Can you work these out from the model? Positions are in its coordinate system, mm. A direction names the side the tool comes from. Give positions to 0.01 mm unless a question says otherwise; leave off trailing zeros. Order: outer loops, then holes, each group sorted by start corner. A loop starts at its lowest first (then second) coordinate and runs counter-clockwise, first axis right, second up. Notation, with made-up numbers: (36.25, -33) - (53.25, -33) arc R8 ccw to (53.25, -20) - close; hole circle Ø6 at (-39.75, 82). An arc over 180 degrees is marked (long way). Answer as a JSON object with one key per item and string values.
```python
from build123d import *

# Parameters (mm, degrees)
BOSS_EXTRUDE1_DEPTH = 12.7
SKETCH2_R           = 1.1303
CUT_EXTRUDE1_DEPTH  = 10
SKETCH3_R           = 3.2639
CUT_EXTRUDE2_DEPTH  = 10


with BuildPart() as part:
    # Sketch1 → Boss-Extrude1 (new body)
    # profile 1 of 4: a face of its own
    with BuildSketch(Plane.XY):
        Polygon((-152.4, 0), (0, 0), (-114.3, -65.991135768), align=None)
        Polygon((-119.404432116, -6.35), (-31.030871047, -6.35), (-29.197783942, -9.525), (-95.477954744, -47.791874454), align=None, mode=Mode.SUBTRACT)
    # profile 2 of 4: a face of its own
    with BuildSketch(Plane.XY):
        Polygon((-165.1, 21.997045256), (-170.599261314, 18.822045256), (-157.899261314, -3.175), (-152.4, 0), align=None)
    # profile 3 of 4: a face of its own
    with BuildSketch(Plane.XY):
        Polygon((-157.899261314, -3.175), (-119.799261314, -69.166135768), (-114.3, -65.991135768), (-152.4, 0), align=None)
    # profile 4 of 4: a face of its own
    with BuildSketch(Plane.XY):
        Polygon((-107.099261314, -91.163181024), (-119.799261314, -69.166135768), (-114.3, -65.991135768), (-101.6, -87.988181024), align=None)
    extrude(amount=BOSS_EXTRUDE1_DEPTH)

    # Sketch2 → Cut-Extrude1 (cut)
    with BuildSketch(Plane(origin=(0, 0, 0), x_dir=(1, 0, 0), z_dir=(0, 1, 0))):
        with Locations(Location((-127, -6.35, 0), (0, 0, 180))):
            Circle(SKETCH2_R)
        with Locations(Location((-25.4, -6.35, 0), (0, 0, 180))):
            Circle(SKETCH2_R)
    extrude(amount=-CUT_EXTRUDE1_DEPTH, mode=Mode.SUBTRACT)

    # Sketch3 → Cut-Extrude2 (cut)
    with BuildSketch(Plane(origin=(-114.3, -65.991135768, 0), x_dir=(0, 0, -1), z_dir=(0.8660254037844342, 0.5000000000000079, 0))):
        with Locations(Location((-6.35, 88.9, 0), (0, 0, 90))):
            Circle(SKETCH3_R)
        with Locations(Location((-6.35, -12.7, 0), (0, 0, 90))):
            Circle(SKETCH3_R)
    extrude(amount=-CUT_EXTRUDE2_DEPTH, mode=Mode.SUBTRACT)


solid = part.part
```
Q1. I'm going to push flat-ended pins straight in: pin 1 Ø1.5 at (y, z) = (-15, 6.5) entering from -X; pin 2 Ø1.5 at (x, z) = (-57.5, 1.5) entering from -Y; pin 3 Ø1.5 at (y, z) = (-29.5, 7.5) entering from -X; pin 4 Ø3 at (x, y) = (-126.5, -64.5) entering from +Z. Where does each tip first touch, or does it pass through?
Recorded:
{"pin 1": "stops at x = -151.51", "pin 2": "stops at y = -33.63", "pin 3": "stops at x = -143.13", "pin 4": "passes through"}
Q2. Which directions (+Z, -Z, +X, -X, +Y, -Y) give clear straight access to the entire face, cutting with the end or side of a thin tool? Please do faces 5 (the face through (-77, 0, 6)), 6 (the face through (-109.45, -74.39, 9.08)), 7 (the face through (-167.811, 20.432, 6.261)), 8 (the face through (-30.127, -7.915, 6.261)).
Recorded:
{"face 5": "+Z, -Z, +X, +Y", "face 6": "+Z, -Z, +X", "face 7": "+Z, -Z, -X, +Y", "face 8": "+Z, -Z"}
Q3. If we section it at B-B, the plane y = -16.5: Please give me the cut outline in (x, z).
Recorded:
{"outline": "(-150.21, 0) - (-113.54, 0) - (-113.54, 12.7) - (-150.21, 12.7) - close; (-41.28, 0) - (-28.58, 0) - (-28.58, 12.7) - (-41.28, 12.7) - close"}
Q4. We'd pull the mould along Z, two halves only. Please class faces 1 (the face through (-110, -26, 0)), 2 (the face through (-111.414, -77.251, 3.454)), 3 (the face through (-160.17, 7.19, 4.36)), 4 (the face through (-56.35, -32.534, 6.261)): released by +Z, released by -Z, zero draft, split by the parting line, or undercut.
Recorded:
{"face 1": "released by -Z", "face 2": "undercut", "face 3": "undercut", "face 4": "zero draft"}
Q5. I need wall thicknesses on L1, parallel to Z at x = -127, y = -7; L2, parallel to Y at x = -108, z = 5.75; L3, parallel to Y at x = -103, z = 2. Which ranges of each line are inside material? Lowest first, please.
Recorded:
{"L1": "z = 0 to 5.22, 7.48 to 12.7", "L2": "y = -89.6 to -80.72, -62.35 to -26.1, -6.35 to 0", "L3": "y = -88.8 to -85.56, -59.47 to -34.76, -6.35 to 0"}
Q6. If we section it at A-A, the plane x = -33: Please give me the cut outline in (y, z), then the cut area to 3 significant figures.
Recorded:
{"outline": "(-19.05, 0) - (-11.72, 0) - (-11.72, 12.7) - (-19.05, 12.7) - close; (-6.35, 0) - (0, 0) - (0, 12.7) - (-6.35, 12.7) - close", "area": "174 mm^2"}
